from build123d import *

# Parameters (mm, degrees)
BOSS_EXTRUDE1_DEPTH = 12
CUT_EXTRUDE2_DEPTH  = 10.5
BOSS_EXTRUDE2_DEPTH = 5
CHAMFER1_SIZE       = 1


with BuildPart() as part:
    # Sketch1 → Boss-Extrude1 (new body)
    with BuildSketch(Plane(origin=(0, 0, 0), x_dir=(1, 0, 0), z_dir=(0, 1, 0))):
        Polygon((-0.788281764, 7.5), (0.788281764, 7.5), (2.330393598, 7.172214011), (3.770656048, 6.530967854), (5.046122736, 5.604287062), (6.101049646, 4.432672033), (6.889331411, 3.067327967), (7.376516334, 1.567926949), (7.541312097, 0), (7.376516334, -1.567926949), (6.889331411, -3.067327967), (6.101049646, -4.432672033), (5.046122736, -5.604287062), (3.770656048, -6.530967854), (2.330393598, -7.172214011), (0.788281764, -7.5), (-0.788281764, -7.5), (-2.330393598, -7.172214011), (-3.770656048, -6.530967854), (-5.046122736, -5.604287062), (-6.101049646, -4.432672033), (-6.889331411, -3.067327967), (-7.376516334, -1.567926949), (-7.541312097, 0), (-7.376516334, 1.567926949), (-6.889331411, 3.067327967), (-6.101049646, 4.432672033), (-5.046122736, 5.604287062), (-3.770656048, 6.530967854), (-2.330393598, 7.172214011), align=None)
    extrude(amount=BOSS_EXTRUDE1_DEPTH)

    # Sketch3 → Cut-Extrude2 (cut)
    with BuildSketch(Plane(origin=(0, 0, 0), x_dir=(-1, 0, 0), z_dir=(0, -1, 0))):
        with BuildLine():
            Line((2.669269563, 1.625), (-2.669269563, 1.625))
            ThreePointArc((-2.669269563, 1.625), (-2.72431184, -1.530931089), (0, -3.125))
            ThreePointArc((0, -3.125), (2.72431184, -1.530931089), (2.669269563, 1.625))
        make_face()
    extrude(amount=-CUT_EXTRUDE2_DEPTH, mode=Mode.SUBTRACT)

    # Sketch4 → Boss-Extrude2 (add)
    with BuildSketch(Plane(origin=(0, 0, 0), x_dir=(-1, 0, 0), z_dir=(0, -1, 0))):
        Polygon((-0.788281764, 7.5), (-2.330393598, 7.172214011), (-3.770656048, 6.530967854), (-5.046122736, 5.604287062), (-6.101049646, 4.432672033), (-6.889331411, 3.067327967), (-7.376516334, 1.567926949), (-7.541312097, 0), (-7.376516334, -1.567926949), (-6.889331411, -3.067327967), (-6.101049646, -4.432672033), (-5.046122736, -5.604287062), (-3.770656048, -6.530967854), (-2.330393598, -7.172214011), (-0.788281764, -7.5), (0.788281764, -7.5), (2.330393598, -7.172214011), (3.770656048, -6.530967854), (5.046122736, -5.604287062), (6.101049646, -4.432672033), (6.889331411, -3.067327967), (7.376516334, -1.567926949), (7.541312097, 0), (7.376516334, 1.567926949), (6.889331411, 3.067327967), (6.101049646, 4.432672033), (5.046122736, 5.604287062), (3.770656048, 6.530967854), (2.330393598, 7.172214011), (0.788281764, 7.5), align=None)
        with BuildLine():
            ThreePointArc((-4, 0), (0, -4), (4, 0))
            ThreePointArc((4, 0), (0, 4), (-4, 0))
        make_face(mode=Mode.SUBTRACT)
    extrude(amount=BOSS_EXTRUDE2_DEPTH)

    # Chamfer1
    chamfer1_edges = [part.edges().sort_by_distance(p)[0] for p in [
        (7.458914215, 12, -0.783963475),
        (7.132923872, 12, -2.317627458),
        (6.495190528, 12, -3.75),
        (5.573586191, 12, -5.018479548),
        (4.408389392, 12, -6.067627458),
        (3.050524823, 12, -6.851590932),
        (-1.559337681, 12, -7.336107006),
        (-3.050524823, 12, -6.851590932),
        (-4.408389392, 12, -6.067627458),
        (-5.573586191, 12, -5.018479548),
        (-6.495190528, 12, -3.75),
        (-7.132923872, 12, -2.317627458),
        (-7.458914215, 12, -0.783963475),
        (-7.458914215, 12, 0.783963475),
        (-7.132923872, 12, 2.317627458),
        (-6.495190528, 12, 3.75),
        (1.559337681, 12, -7.336107006),
        (-5.573586191, 12, 5.018479548),
        (-4.408389392, 12, 6.067627458),
        (-3.050524823, 12, 6.851590932),
        (-1.559337681, 12, 7.336107006),
        (0, 12, 7.5),
        (1.559337681, 12, 7.336107006),
        (3.050524823, 12, 6.851590932),
        (4.408389392, 12, 6.067627458),
        (5.573586191, 12, 5.018479548),
        (6.495190528, 12, 3.75),
        (0, 12, -7.5),
        (7.132923872, 12, 2.317627458),
        (7.458914215, 12, 0.783963475),
    ]]
    chamfer(chamfer1_edges, length=CHAMFER1_SIZE)


solid = part.part
The listing builds one solid part. Answer for the finished solid, in the listing's coordinates (mm). Round coordinates to 2 decimals unless told otherwise and drop trailing zeros. Write each loop counter-clockwise with the first axis right and the second up, starting at its lowest first coordinate (ties: lowest second). Pieces come first, ordered by that corner, then holes. Notation, with made-up numbers: (7.5, 67) - (11.5, 67) arc R20 cw to (11.5, 77) - close; hole circle Ø6 at (-18, -4.5). An arc over 180 degrees is marked (long way). Use a Markdown table: item, result. Add a question column.
1. The part is cut by section C-C (z = -2.25). Write down the section's boundary in (x, y), and give its area (3 significant figures).
2. Flat-ended cylindrical pins translate along their axes: P1, Ø8, axis at x = 2, y = 5.5, coming from the -Z side; P2, Ø3, axis at x = 4.5, y = 8, coming from the +Z side; P3, Ø1, axis at x = 4, y = 5.5, coming from the +Z side; P4, Ø2.5, axis at x = 1, z = 1.5, coming from the -Y side. Find the tip coordinate at first contact, or state that the pin passes through.
3. Consider line 1 (Z direction, x = 0, y = -2.75); line 2 (X direction, y = 3.5, z = 1.5); line 3 (Y direction, x = -0.75, z = 1). Determine where each line is inside the solid, lowest interval first.
4. For a pull along X with two mould halves and no side action, classify faces 1 (the face through (-2.86, 11.49, -6.4)), 2 (the face through (0, 10.5, 1)), 3 (the face through (4.42, 3.11, 6.06)) as +X half, -X half, draft (parallel to the pull), parting line (faces both ways), or undercut.
Reported:
| question | item | result |
|---|---|---|
| 1 | outline | (-7.15, -5) - (-3.31, -5) - (-3.31, 0) - (3.31, 0) - (3.31, -5) - (7.15, -5) - (7.15, 11) - (6.1, 12) - (-6.1, 12) - (-7.15, 11) - close |
| 1 | area | 209 mm^2 |
| 2 | P1 | z = -7.5 |
| 2 | P2 | z = 6.87 |
| 2 | P3 | z = 6.65 |
| 2 | P4 | y = 10.5 |
| 3 | line 1 | -7.5 to -4, 4 to 7.5 |
| 3 | line 2 | -7.38 to -2.74, 2.74 to 7.38 |
| 3 | line 3 | 10.5 to 12 |
| 4 | face 1 | -X half |
| 4 | face 2 | undercut |
| 4 | face 3 | +X half |
